Autodesk Fusion 360 part; units mm, degrees
sketch "スケッチ1" plane through (0, 0, 0) normal (0, 0, 1) x (1, 0, 0)
  line L0 (0, 0) -> (18.1957, 0)
  line L1 (18.1957, 0) -> (18.1957, 13.2439)
  line L2 (18.1957, 13.2439) -> (0, 13.2439)
  line L3 (0, 13.2439) -> (0, 0)
  line L4 (0, 0) -> (-13.9996, 0)
  line L5 (-13.9996, 0) -> (-13.9996, 13.2439)
  line L6 (-13.9996, 13.2439) -> (0, 13.2439)
  line L7 (0, 13.2439) -> (0, 0)
  circle A0 centre (-7.0436, 4.9) radius 2
  circle A1 centre (7.0436, 4.9) radius 2
  circle A2 centre (0, 9) radius 2
  circle A3 centre (14.2957, 2.8) radius 3
  circle A4 centre (-7.0436, 4.9) radius 2.5
  circle A5 centre (7.0436, 4.9) radius 2.5
  circle A6 centre (0, 9) radius 2.3
  circle A7 centre (0, 9) radius 1.7
  line L8 (-7, 1.5003) -> (-7, 0)
  line L9 (7, 1.5003) -> (7, 0)
  circle A8 centre (-7.0436, 4.9) radius 3.4
  circle A9 centre (0, 9) radius 2.9
  line L10 (-7.0436, 4.9) -> (0, 9)
  line L11 (0, 9) -> (7.0436, 4.9)
  line L12 (7.0436, 4.9) -> (14.2957, 2.8)
  circle A10 centre (7.0436, 4.9) radius 3.4
  circle A11 centre (14.2957, 2.8) radius 3.9
  line L13 (-4.6, 2.5359) -> (-4.6, 0)
  line L14 (4.6, 2.5359) -> (4.6, 0)
  line L15 (-9.4, 2.449) -> (-9.4, 0)
  line L16 (9.4, 2.449) -> (9.4, 0)
  line L17 (-3.6906, 5.4633) -> (-1.678, 6.6348)
  line L18 (1.678, 6.6348) -> (3.6906, 5.4633)
  line L19 (-4.898, 7.5375) -> (-2.8854, 8.709)
  line L20 (2.8854, 8.709) -> (4.898, 7.5375)
  line L21 (10.3149, 5.8267) -> (11.4731, 5.4913)
  line L22 (9.3136, 2.3687) -> (10.4718, 2.0333)
  line L23 (0, 0) -> (18.1957, 0)
  line L24 (18.1957, 0) -> (18.1957, -2.0683)
  line L25 (18.1957, -2.0683) -> (0, -2.0683)
  line L26 (-13.9996, 0) -> (0, 0)
  line L27 (0, -2.0683) -> (-13.9996, -2.0683)
  line L28 (-13.9996, -2.0683) -> (-13.9996, 0)
  line L29 (-12.3, 6.4) -> (-12.3, 10)
  line L30 (-12.3, 10) -> (-8.7, 10)
  line L31 (-8.7, 10) -> (-8.7, 7.8692)
  line L32 (-12.3, 6.4) -> (-10.0948, 6.4)
  line L33 (-5.5, 1.65) -> (-8.5, 1.65)
  line L34 (-8.5, 1.65) -> (-8.5, 0.4)
  line L35 (-8.5, 0.4) -> (-5.5, 0.4)
  line L36 (-5.5, 0.4) -> (-5.5, 1.65)
  line L37 (-5.5, 1.65) -> (-8.5, 0.4) construction
  line L38 (-8.5, 1.65) -> (-5.5, 0.4) construction
  line L39 (8.5, 1.65) -> (5.5, 1.65)
  line L40 (5.5, 1.65) -> (5.5, 0.4)
  line L41 (5.5, 0.4) -> (8.5, 0.4)
  line L42 (8.5, 0.4) -> (8.5, 1.65)
  line L43 (8.5, 1.65) -> (5.5, 0.4) construction
  line L44 (5.5, 1.65) -> (8.5, 0.4) construction
  arc A12 (-12.3, 9.4) -> (-9.3, 6.4) centre (-9.3, 9.4) ccw
  point P0 (-7, 1.5003)
  point P1 (7, 1.5003)
  point P2 (-10.5, 10)
  point P3 (-7, 1.025)
  point P4 (7, 1.025)
  dimension "d4" = 4
  dimension "d5" = 4.9
  dimension "d6" = 8.15
  dimension "d7" = 4
  dimension "d10" = 6
  dimension "d16" = 2.8
  dimension "d18" = 9
  dimension "d19" = 5
  dimension "d21" = 7.55
  dimension "d26" = 4.6
  dimension "d34" = 3.4
  dimension "d41" = 7
  dimension "d45" = 5.8
  dimension "d51" = 1.2
  dimension "d52" = 4.8
  dimension "d54" = 1.8
  dimension "d57" = 6.8
  dimension "d76" = 7.8
  dimension "d86" = 10.5
  dimension "d87" = 3.6
  dimension "d88" = 10
  dimension "d92" = 3
  dimension "d93" = 0.4
  dimension "d94" = 1.25
  dimension "d96" = 3.6
  dimension "d97" = 3
extrude "押し出し1" add sketch "スケッチ1" along normal blind 3 contours L0 L9 A10 L14 L23 L39 L40 L41 | L3 L7 A6 A9 L10 | L3 L7 A6 A9 L11 | L4 L8 A8 L13 L26 L33 L35 L36 | L0 L9 A10 L16 L22 L23 L39 L41 L42 | A5 L11 L12 A10 L39 | A8 A9 L10 L17 | A9 L11 A10 L18 | L4 L8 A8 L15 L26 L33 L34 L35 | A8 L33 | L3 L7 A6 A9 L10 | L3 L7 A6 A9 L11 | A8 A9 L10 L19 | A9 L11 A10 L20 | L0 A3 L12 A11 L23 | L0 A3 A11 L23 | A10 L16 L22 | L12 A10 A11 L16 L22 | A5 L11 L12 A10 | L0 A3 L12 A11 L23 | L12 A10 A11 L21 | A8 L29 L30 L31 A12 picked at (-7.0875, 1.9012)
extrude "押し出し2" add sketch "スケッチ1" along normal blind 0.5 contours A4 | A1 A5 L11 L12 | A1 A5 L11 L12
extrude "押し出し5" add sketch "スケッチ1" against normal blind 2.3 from surface at 3 contours L3 L7 A2 A6 L10 | L3 L7 A2 A6 L11 | L3 L7 A2 A6 L10 | L3 L7 A2 A6 L11
sketch "スケッチ2" plane through (0, 0, 0) normal (0, -1, 0) x (1, 0, 0)
  line L0 (-7, 0) -> (-7, 3)
  line L1 (7, 0) -> (7, 3)
  circle A0 centre (-7, 1.5) radius 0.8
  circle A1 centre (7, 1.5) radius 0.8
  line L2 (9.4, 0) -> (9.4, 3)
  line L3 (4.6, 3) -> (4.6, 0)
  line L4 (-4.6, 3) -> (-9.4, 3)
  line L5 (4.6, 0) -> (9.4, 0)
  line L6 (-4.6, 0) -> (-4.6, 3)
  line L7 (-9.4, 3) -> (-9.4, 0)
  line L8 (9.4, 3) -> (4.6, 3)
  line L9 (-9.4, 0) -> (-4.6, 0)
  point P0 (7, 0)
  dimension "d42" = 1.6
extrude "押し出し7" cut sketch "スケッチ2" against normal blind 3 contours L0 A0 | L0 A0 | L1 A1 | L1 A1
extrude "押し出し8" add sketch "スケッチ1" against normal blind 0.3 from surface at 1 contours L3 L7 A2 A7 L10 | L3 L7 A2 A7 L11 | L3 L7 A2 A7 L10 | L3 L7 A2 A7 L11
sketch "スケッチ6" plane through (0, 10, 0) normal (0, 1, 0) x (-1, 0, 0)
  line L0 (8.7, 0) -> (12.3, 0)
  line L1 (12.3, 0) -> (12.3, 3)
  line L2 (12.3, 3) -> (8.7, 3)
  line L3 (8.7, 3) -> (8.7, 0)
  line L4 (10.5, 3) -> (10.5, 0)
  circle A0 centre (10.5, 1.5) radius 0.75
  dimension "d89" = 1.5
extrude "押し出し12" cut sketch "スケッチ6" against normal blind 2.6 contours L4 A0 | L4 A0
equation "d5 = 6.5 mm - 0.6 mm - 1.0 mm"
equation "d6 = 6.15 mm + 1.95 mm + 0.05 mm"
equation "d16 = ( 7.8 / 2 ) * 1 mm - 0.6 mm - 0.5 mm"
equation "d21 = 6.15 mm + 1.35 mm + 0.05 mm"
Here's how the part is built. I have some questions about the finished solid (model axes, mm). A direction names the side the tool comes from. Coordinates: 2 decimals unless noted, no trailing zeros. Write each loop counter-clockwise with the first axis right and the second up, starting at its lowest first coordinate (ties: lowest second). Pieces come first, ordered by that corner, then holes.
Item 1: If we mould it in two halves opening along X, with no side actions, what happens to faces 1 (the flat face through (-6, 0, 1)), 2 (the flat face through (-9.4, 1, 1)), 3 (the cylindrical face through (-9.75, 8.72, 1.53))? For each: +X half, -X half, draft (parallel to the pull), parting line (faces both ways), or undercut.
Item 2: I want a section at A-A on x = 0. Write out the boundary of the cut face in (y, z).
Item 3: Will these pins go through, and if not, where does the flat tip stop? pin 1 (0.6 mm diameter, centred on y = 1, z = 2, fed in from -X); pin 2 (1 mm diameter, centred on x = 0.5, y = 4, fed in from +Z); pin 3 (4.5 mm diameter, centred on x = 0, y = 9, fed in from -Z); pin 4 (1.5 mm diameter, centred on x = -9.5, z = 1, fed in from +Y).
Item 4: If I drill on line 1 (X direction, y = 4.75, z = 2.6); line 2 (Y direction, x = 0, z = 0.55); line 3 (Y direction, x = -7, z = 2.6), over which ranges is the centre line in solid material (lowest first)?
Item 5: I want a section at B-B on y = 1. Write out the boundary of the cut face in (x, z).
Item 6: I want a section at C-C on x = 7. Write out the boundary of the cut face in (y, z), and give its area (3 significant figures).
Item 7: On a 3-axis mill with a long thin cutter (end or side, diameter ignored), from which of +Z, -Z, +X, -X, +Y, -Y can I reach the whole of each face in a straight line? I mean faces 4 (the cylindrical face through (-7.8, 0.2, 1.5)), 5 (the cylindrical face through (-0.3, 6.72, 0.35)), 6 (the flat face through (4.6, 1, 1)). Say none if no direction works.
Item 8: I want a section at D-D on y = 9. Write out the boundary of the cut face in (x, z), and give its area (3 significant figures).
Findings below:
1. face 1: draft
1. face 2: -X half
1. face 3: undercut
2. outline: (6.1, 0) - (6.7, 0) - (6.7, 0.7) - (7.3, 0.7) - (7.3, 1) - (7, 1) - (7, 3) - (6.1, 3) - close; (10.7, 0.7) - (11.3, 0.7) - (11.3, 0) - (11.9, 0) - (11.9, 3) - (11, 3) - (11, 1) - (10.7, 1) - close
3. pin 1: stops at x = -9.4
3. pin 2: passes through
3. pin 3: stops at z = 0.7
3. pin 4: stops at y = 10
4. line 1: x = -10.44 to -9.54, -4.55 to -3.65, 3.65 to 4.55, 9.54 to 12.02, 16.58 to 17.67
4. line 2: y = 6.1 to 6.7, 11.3 to 11.9
4. line 3: y = 0 to 0.4, 1.65 to 2.4, 7.4 to 8.3
5. outline: (-9.4, 0) - (-8.5, 0) - (-8.5, 3) - (-9.4, 3) - close; (-5.5, 0) - (-4.6, 0) - (-4.6, 3) - (-5.5, 3) - close; (4.6, 0) - (5.5, 0) - (5.5, 3) - (4.6, 3) - close; (8.5, 0) - (9.4, 0) - (9.4, 3) - (8.5, 3) - close; (10.84, 0) - (11.9, 0) - (11.9, 3) - (10.84, 3) - close; (16.7, 0) - (17.76, 0) - (17.76, 3) - (16.7, 3) - close
6. outline: (0, 0) - (0.4, 0) - (0.4, 0.7) - (0, 0.7) - close; (0, 2.3) - (0.4, 2.3) - (0.4, 3) - (0, 3) - close; (1.65, 0) - (2.9, 0) - (2.9, 0.5) - (2.4, 0.5) - (2.4, 0.7) - (1.65, 0.7) - close; (1.65, 2.3) - (2.4, 2.3) - (2.4, 3) - (1.65, 3) - close; (6.9, 0) - (8.3, 0) - (8.3, 3) - (7.4, 3) - (7.4, 0.5) - (6.9, 0.5) - close
6. area: 4.81 mm2
7. face 4: -Y
7. face 5: -Z
7. face 6: +Z, -Z, -Y
8. outline: (-12.27, 0) - (-8.7, 0) - (-8.7, 3) - (-12.27, 3) - close; (-2.9, 0) - (-2.3, 0) - (-2.3, 0.7) - (-1.7, 0.7) - (-1.7, 1) - (-2, 1) - (-2, 3) - (-2.9, 3) - close; (1.7, 0.7) - (2.3, 0.7) - (2.3, 0) - (2.9, 0) - (2.9, 3) - (2, 3) - (2, 1) - (1.7, 1) - close; hole circle Ø1.5 at (-10.5, 1.5)
8. area: 14.1 mm2
